Verification items for this drawing (mm, ordinates from the low corner). Give positions to 0.01 mm unless a question says otherwise; leave off trailing zeros. Loops run counter-clockwise (first coordinate to the right, second up) from the corner with the lowest first, then second, coordinate; pieces in that order, holes last. Notation, with made-up numbers: M 16.25,83 L 60.25,83 A23 cw 60.25,98 Z; hole C 13,45 d6. An arc over 180 degrees is marked long. Answer in a Markdown table with one row per item.
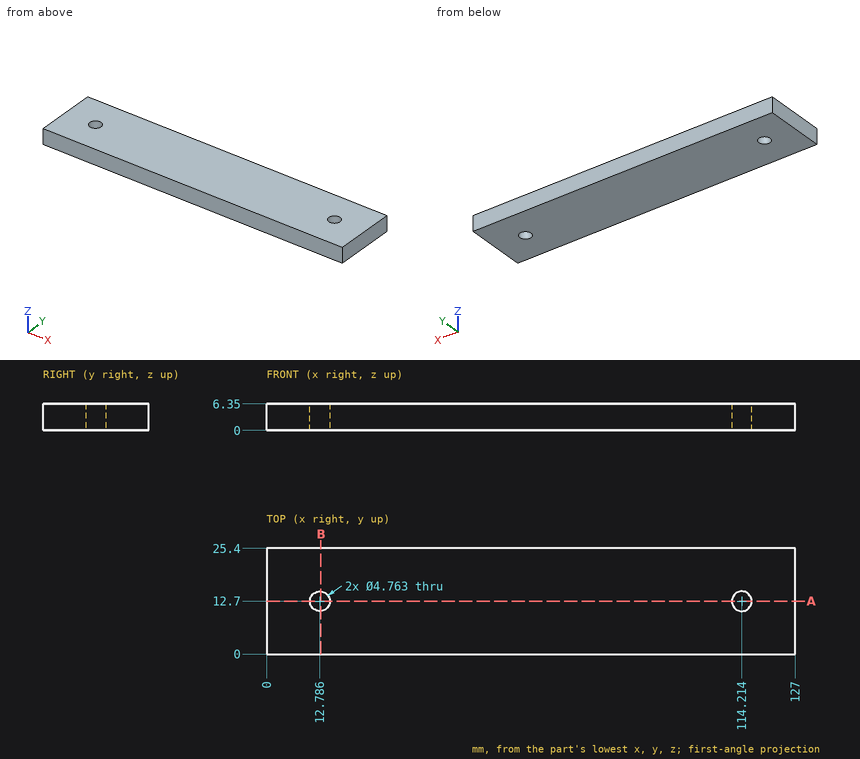
Item 1: Sectioned sample at B-B (x = 13). Record the cut outline in (y, z).
Reported:
| item | result |
|---|---|
| outline | M 0,0 L 10.33,0 L 10.33,6.35 L 0,6.35 Z; M 15.07,0 L 25.4,0 L 25.4,6.35 L 15.07,6.35 Z |
Item 2: Sectioned sample at A-A (y = 12.7). State how many separate pieces and enclosed holes the cut face has, and give its area (3 significant figures).
Reported:
| item | result |
|---|---|
| separate pieces | 3 |
| enclosed holes | 0 |
| area | 746 mm^2 |
Item 3: Scan lines: L1, parallel to X at y = 12.5, z = 2.25; L2, parallel to X at y = 14.75, z = 3.25 (1 decimal); L3, parallel to Y at x = 114.5, z = 0.5 (1 decimal). Record each from-to range of solid material in increasing order. Write a range as [from, to].
Reported:
| item | result |
|---|---|
| L1 | x = [0, 10.41], [15.16, 111.84], [116.59, 127] |
| L2 | x = [0, 11.6], [14, 113], [115.4, 127] |
| L3 | y = [0, 10.3], [15.1, 25.4] |
